Work out the finished part from the listing and answer in its coordinate system (mm). A direction names the side the tool comes from. Coordinates: 2 decimals unless noted, no trailing zeros. Order: outer loops, then holes, each group sorted by start corner. A loop starts at its lowest first (then second) coordinate and runs counter-clockwise, first axis right, second up. Notation, with made-up numbers: (42, 66.5) -> (94, 66.5) arc R26 cw to (94, 97.5) -> close; hole circle Ø11 at (-5.75, -22). An arc over 180 degrees is marked (long way). Use one line per item in the form item = value.
Autodesk Inventor part; units mm, degrees
ref_plane "YZ Plane" through (0, 0, 0) normal (1, 0, 0) x (0, 1, 0)
ref_plane "XZ Plane" through (0, 0, 0) normal (0, 1, 0) x (-1, 0, 0)
ref_plane "XY Plane" through (0, 0, 0) normal (0, 0, 1) x (1, 0, 0)
sketch "Náčrt1" plane through (0, 0, 0) normal (0, 0, 1) x (1, 0, 0)
  line L0 (0, 0) -> (40, 0)
  line L1 (40, 0) -> (40, 40)
  line L2 (40, 40) -> (30, 40)
  line L3 (30, 40) -> (30, 30)
  line L4 (30, 30) -> (10, 30)
  line L5 (10, 30) -> (10, 40)
  line L6 (10, 40) -> (0, 40)
  line L7 (0, 40) -> (0, 0)
  dimension "d0" = 40
  dimension "d1" = 40
  dimension "d2" = 10
  dimension "d3" = 10
  dimension "d4" = 20
  dimension "d5" = 10
  dimension "d6" = 10
extrude "Vysunutí1" add sketch "Náčrt1" against normal blind 60
sketch "Náčrt2" plane through (0, 0, 0) normal (0, 0, 1) x (1, 0, 0)
  line L0 (40, 0) -> (0, 0)
  line L1 (40, 0) -> (40, 20)
  line L2 (40, 0) -> (40, 40)
  line L3 (40, 20) -> (20, 20)
  line L4 (20, 20) -> (20, 0)
  line L5 (20, 0) -> (40, 0)
  dimension "d11" = 20
  dimension "d12" = 20
extrude "Vysunutí2" cut sketch "Náčrt2" against normal blind 25
sketch "Náčrt3" plane through (0, 0, 0) normal (-1, 0, 0) x (0, 0, 1)
  line L0 (0, 40) -> (0, 0)
  line L1 (-25, 0) -> (0, 0)
  line L2 (0, 0) -> (-25, 0)
  line L3 (0, 20) -> (-25, 0)
  line L4 (0, 0) -> (0, 20)
extrude "Vysunutí3" cut sketch "Náčrt3" against normal blind 25
properties part number "5"
(1) Straight lines are drawn through the part: line 1 along X through (y, z) = (33.5, -37); line 2 along Y through (x, z) = (21, -35.5); line 3 along Z through (x, y) = (26.5, 18.5). For each, find the intervals that lie inside material, in ascending order.
Data:
line_1 = 0 to 10, 30 to 40
line_2 = 0 to 30
line_3 = -60 to -25
(2) Section C-C on x = 16 is taken. Write down the section's boundary in (y, z).
Data:
outline = (0, -60) -> (30, -60) -> (30, 0) -> (20, 0) -> (0, -25) -> close
(3) The mould has two halves that part along X. Classify faces 4 (the flat face through (30, 20, -12)), 5 (the flat face through (20, 15, -18)), 6 (the flat face through (20, 30, -30)): released by +X, released by -X, zero draft, split by the parting line, or undercut.
Data:
face_4 = zero draft
face_5 = released by +X
face_6 = undercut
(4) Section B-B on y = 14 is taken. Write down the section's boundary in (x, z).
Data:
outline = (0, -60) -> (40, -60) -> (40, -25) -> (20, -25) -> (20, -7.5) -> (0, -7.5) -> close
(5) Which of the six approach directions +Z, -Z, +X, -X, +Y, -Y give full straight-line access (tool end or side, diameter ignored) to faces 1 (the flat face through (0, 20, -30)), 2 (the flat face through (30, 10, -25)), 3 (the flat face through (10, 35, -30))?
Data:
face_1 = +Z, -Z, -X, +Y, -Y
face_2 = +Z, +X, -Y
face_3 = +Z, -Z, +Y
(6) Each of these flat-tipped pins is pushed along its axis until it touches: P1, Ø4, axis at x = 16, y = 15, coming from the +Z side; P2, Ø1.5, axis at x = 35.5, y = 31.5, coming from the +Z side; P3, Ø2, axis at x = 19.5, z = -37.5, coming from the +Y side; P4, Ø4, axis at x = 35.5, z = -17, coming from the -Y side. Where does it stop, or does it pass through?
Data:
P1 = -3.75
P2 = 0
P3 = 30
P4 = 20
(7) Section D-D on z = -5 is taken. Write down the section's boundary in (x, y), plus the area to 3 significant figures.
Data:
outline = (0, 16) -> (20, 16) -> (20, 20) -> (40, 20) -> (40, 40) -> (30, 40) -> (30, 30) -> (10, 30) -> (10, 40) -> (0, 40) -> close
area = 680 mm²
(8) Section A-A on z = -37.5 is taken. Write down the section's boundary in (x, y).
Data:
outline = (0, 0) -> (40, 0) -> (40, 40) -> (30, 40) -> (30, 30) -> (10, 30) -> (10, 40) -> (0, 40) -> close
